The listing builds one solid part. Answer for the finished solid, in the listing's coordinates (mm). A direction names the side the tool comes from. Coordinates: 2 decimals unless noted, no trailing zeros. Order: outer loops, then holes, each group sorted by start corner. A loop starts at its lowest first (then second) coordinate and runs counter-clockwise, first axis right, second up. Notation, with made-up numbers: M -27.75,-36.75 L -4.75,-36.75 A11 ccw -4.75,-19.75 Z; hole C 61,1 d10. An arc over 180 degrees is marked long. One line per item, written item: value. Start each with the question number.
Q1. The part is cut by section B-B on x = 0. Give the number of separate pieces and of enclosed holes in the cut face, then the cut area to 3 significant figures.
Q2. The part is cut by section D-D on z = 11. Give the vertices of the cut face in (x, y), then the cut area to 3 significant figures.
Q3. The part is cut by section A-A on y = 0. Give the vertices of the cut face in (x, z), then the cut area to 3 significant figures.
Q4. Straight lines are drawn through the part: line 1 along Y through (x, z) = (0, 27); line 2 along Y through (x, z) = (0, 31.15); line 3 along Y through (x, z) = (0, 27.85). For each, find the intervals that lie inside material, in ascending order. Write a range as [from, to].
Q5. Each of these flat-tipped pins is pushed along its axis until it touches: pin 1 Ø7 at (x, y) = (0, -14) entering from +Z; pin 2 Ø1.5 at (y, z) = (28, 22.5) entering from -X; pin 3 Ø1.5 at (x, z) = (-39, 21.5) entering from -Y; pin 4 Ø5 at (y, z) = (-26.5, 14.5) entering from +X. Where does it stop, or does it pass through?
Q6. The part is cut by section C-C on z = 3. Give the vertices of the cut face in (x, y), then the cut area to 3 significant figures.
Q7. Determine the mould class of faces 1 (the flat face through (26, 0, 28.385)), 2 (the cylindrical face through (5.5, 24.9, 30.4)), 3 (the flat face through (0, -6, 28.385)) for opening direction X: pulls with the +X half, pulls with the -X half, needs draft (parallel to the pull), parting line crosses it, or undercut.
Q8. For faces 4 (the flat face through (-6, 0, 25.385)), 5 (the cylindrical face through (-22.4, -7.1, 30.4)), 6 (the cylindrical face through (-0.488, -16.196, 26.906)), determine the directions among +Z, -Z, +X, -X, +Y, -Y from which every point of the face is accessible in a straight line to the end or side of a thin tool.
```python
from build123d import *

# Parameters (mm, degrees)
F2_R     = 3.75
F2_R_2   = 2.25
F3_DEPTH = 25
F4_R     = 5.5
F5_DEPTH = 1


with BuildPart() as f1:
    # F0 (on Front) → F1 (revolve)
    with BuildSketch(Plane.XZ):
        Polygon((-23.5, 28.38492), (-23.5, 32.384921), (-25.5, 32.384921), (-25.5, 28.38492), (-31.5, 28.38492), (-52.571308, -5.61508), (-49.011947, -5.566755), (-29.829821, 25.38492), (0, 25.38492), (0, 28.38492), align=None)
    revolve(axis=Axis((0, 0, 26.88492), (0, 0, 1)))

    # F2 (on face) → F3 (cut)
    with BuildSketch(Plane.XY.offset(28.38492)):
        Circle(F2_R)
        with Locations((0, -14)):
            Circle(F2_R_2)
        with Locations((0, 14)):
            Circle(F2_R_2)
    extrude(amount=-F3_DEPTH, mode=Mode.SUBTRACT)

    # F4 (on face) → F5 (cut)
    with BuildSketch(Plane.XY.offset(28.38492)):
        Circle(F4_R)
    extrude(amount=-F5_DEPTH, mode=Mode.SUBTRACT)


solid = f1.part
```
Output:
1. separate pieces: 4
1. enclosed holes: 0
1. area: 376 mm^2
2. outline: C 0,0 d84.55; hole C 0,0 d77.49
2. area: 898 mm^2
3. outline: M -52.57,-5.62 L -49.01,-5.57 L -29.83,25.38 L -3.75,25.38 L -3.75,27.38 L -5.5,27.38 L -5.5,28.38 L -23.5,28.38 L -23.5,32.38 L -25.5,32.38 L -25.5,28.38 L -31.5,28.38 Z; M 3.75,25.38 L 29.83,25.38 L 49.01,-5.57 L 52.57,-5.62 L 31.5,28.38 L 25.5,28.38 L 25.5,32.38 L 23.5,32.38 L 23.5,28.38 L 5.5,28.38 L 5.5,27.38 L 3.75,27.38 Z
3. area: 403 mm^2
4. line 1: y = [-32.36, -16.25], [-11.75, -3.75], [3.75, 11.75], [16.25, 32.36]
4. line 2: y = [-25.5, -23.5], [23.5, 25.5]
4. line 3: y = [-31.83, -16.25], [-11.75, -5.5], [5.5, 11.75], [16.25, 31.83]
5. pin 1: stops at z = 28.38
5. pin 2: stops at x = -22.46
5. pin 3: passes through
5. pin 4: stops at x = 32.95
6. outline: C 0,0 d94.46; hole C 0,0 d87.41
6. area: 1,010 mm^2
7. face 1: needs draft
7. face 2: parting line crosses it
7. face 3: undercut
8. face 4: -Z
8. face 5: +Z
8. face 6: +Z, -Z
